from build123d import *

# Parameters (mm, degrees)
F0_R     = 1.45
F0_R_2   = 1.65
F0_R_3   = 2.25
F1_DEPTH = 4


with BuildPart() as f1:
    # F0 (on Top) → F1 (new body)
    with BuildSketch(Plane.XY):
        with BuildLine():
            Line((-1.25, 22.5), (-1.25, 49.5))
            ThreePointArc((-1.25, 49.5), (-5.75, 54), (-10.25, 49.5))
            Line((-10.25, 49.5), (-10.25, 22.5))
            Line((-10.25, 22.5), (-18.5, 22.5))
            ThreePointArc((-18.5, 22.5), (-21.328427, 21.328427), (-22.5, 18.5))
            Line((-22.5, 18.5), (-22.5, -18.5))
            ThreePointArc((-22.5, -18.5), (-21.328427, -21.328427), (-18.5, -22.5))
            Line((-18.5, -22.5), (9, -22.5))
            Line((9, -22.5), (9, -30.75))
            ThreePointArc((9, -30.75), (9.292893, -31.457107), (10, -31.75))
            Line((10, -31.75), (16.5, -31.75))
            Line((16.5, -31.75), (16.5, -22.5))
            Line((16.5, -22.5), (18.5, -22.5))
            ThreePointArc((18.5, -22.5), (21.328427, -21.328427), (22.5, -18.5))
            Line((22.5, -18.5), (22.5, 18.5))
            ThreePointArc((22.5, 18.5), (21.328427, 21.328427), (18.5, 22.5))
            Line((18.5, 22.5), (-1.25, 22.5))
        make_face()
        with Locations((-13.5, -18.5)):
            Circle(F0_R, mode=Mode.SUBTRACT)
        with Locations((-8.5, -9.5)):
            Circle(F0_R_2, mode=Mode.SUBTRACT)
        with Locations((-8.5, 9.5)):
            Circle(F0_R_2, mode=Mode.SUBTRACT)
        with Locations((13.5, -26.5)):
            Circle(F0_R_2, mode=Mode.SUBTRACT)
        with Locations((13.5, -18.5)):
            Circle(F0_R, mode=Mode.SUBTRACT)
        with Locations((8.5, -9.5)):
            Circle(F0_R_2, mode=Mode.SUBTRACT)
        with Locations((8.5, 9.5)):
            Circle(F0_R_2, mode=Mode.SUBTRACT)
        with Locations((-5.75, 49.5)):
            Circle(F0_R_3, mode=Mode.SUBTRACT)
    extrude(amount=-F1_DEPTH)


solid = f1.part
Here's how the part is built. I have some questions about the finished solid (model axes, mm). A direction names the side the tool comes from. Give positions to 0.01 mm unless a question says otherwise; leave off trailing zeros. Loops run counter-clockwise (first coordinate to the right, second up) from the corner with the lowest first, then second, coordinate; pieces in that order, holes last. Notation, with made-up numbers: (-35.5, -28) -> (-27.5, -28) arc R18 ccw to (-27.5, 5) -> close; hole circle Ø6 at (61, -20.75). An arc over 180 degrees is marked (long way). Answer as a JSON object with one key per item and string values. Group by question number.
Item 1: Imagine slicing it at A-A on x = -13.5. Write out the boundary of the cut face in (y, z), then the cut area to 3 significant figures.
Item 2: Thinking about a two-plate mould opening in X: for faces 1 (the cylindrical face through (-6.04, 51.73, -1.97)), 2 (the cylindrical face through (8.1, 7.9, -2)), 3 (the flat face through (0, 2, -4)), 4 (the flat face through (9, -27, -2)), which applies, pulls with the +X half, pulls with the -X half, needs draft (parallel to the pull), parting line crosses it, or undercut?
Item 3: Imagine slicing it at B-B on y = 9.5. Write out the boundary of the cut face in (x, z).
Item 4: On a 3-axis mill with a long thin cutter (end or side, diameter ignored), from which of +Z, -Z, +X, -X, +Y, -Y can I reach the whole of each face in a straight line? I mean faces 5 (the flat face through (17, -22.5, -2)), 6 (the flat face through (-10.25, 36, -2)), 7 (the cylindrical face through (-21.359, -21.297, -1.972)), 8 (the flat face through (9, 22.5, -2)). Say none if no direction works.
Item 5: Imagine slicing it at C-C on z = -1. Give the number of separate pieces and of enclosed holes in the cut face, then the cut area to 3 significant figures.
Item 6: Will these pins go through, and if not, where does the flat tip stop? pin 1 (2 mm diameter, centred on x = -13.5, z = -2.5, fed in from +Y); pin 2 (1.2 mm diameter, centred on x = -1.5, z = -1, fed in from -Y); pin 3 (1.2 mm diameter, centred on y = -27.5, z = -2.5, fed in from -X); pin 4 (4 mm diameter, centred on x = 13.5, y = -18.5, fed in from -Z).
Item 7: I need wall thicknesses on L1, parallel to Y at x = 8.5, z = -2.1; L2, parallel to Y at x = -8.5, z = -1.4; L3, parallel to Y at x = -5.75, z = -1.9. Which ranges of each line are inside material? Lowest first, please.
Item 8: Imagine slicing it at D-D on x = -5.75. Write out the boundary of the cut face in (y, z), then the cut area to 3 significant figures.
Answer list:
{
 "1": {"outline": "(-22.5, -4) -> (-19.95, -4) -> (-19.95, 0) -> (-22.5, 0) -> close; (-17.05, -4) -> (22.5, -4) -> (22.5, 0) -> (-17.05, 0) -> close", "area": "168 mm2"},
 "2": {"face 1": "undercut", "face 2": "undercut", "face 3": "needs draft", "face 4": "pulls with the -X half"},
 "3": {"outline": "(-22.5, -4) -> (-10.15, -4) -> (-10.15, 0) -> (-22.5, 0) -> close; (-6.85, -4) -> (6.85, -4) -> (6.85, 0) -> (-6.85, 0) -> close; (10.15, -4) -> (22.5, -4) -> (22.5, 0) -> (10.15, 0) -> close"},
 "4": {"face 5": "+Z, -Z, +X, -Y", "face 6": "+Z, -Z, -X, +Y", "face 7": "+Z, -Z, -X, -Y", "face 8": "+Z, -Z, +X, +Y"},
 "5": {"separate pieces": "1", "enclosed holes": "8", "area": "2,280 mm2"},
 "6": {"pin 1": "stops at y = 22.5", "pin 2": "stops at y = -22.5", "pin 3": "stops at x = 9", "pin 4": "stops at z = -4"},
 "7": {"L1": "y = -22.5 to -11.15, -7.85 to 7.85, 11.15 to 22.5", "L2": "y = -22.5 to -11.15, -7.85 to 7.85, 11.15 to 53.06", "L3": "y = -22.5 to 47.25, 51.75 to 54"},
 "8": {"outline": "(-22.5, -4) -> (47.25, -4) -> (47.25, 0) -> (-22.5, 0) -> close; (51.75, -4) -> (54, -4) -> (54, 0) -> (51.75, 0) -> close", "area": "288 mm2"}
}
